Geometry check sheet. Reference: the model listing, model coordinates, mm. Face numbers are marked on the shaded views. A direction names the side the tool comes from. Coordinates: 2 decimals unless noted, no trailing zeros. One line per question, with ' | ' between items.
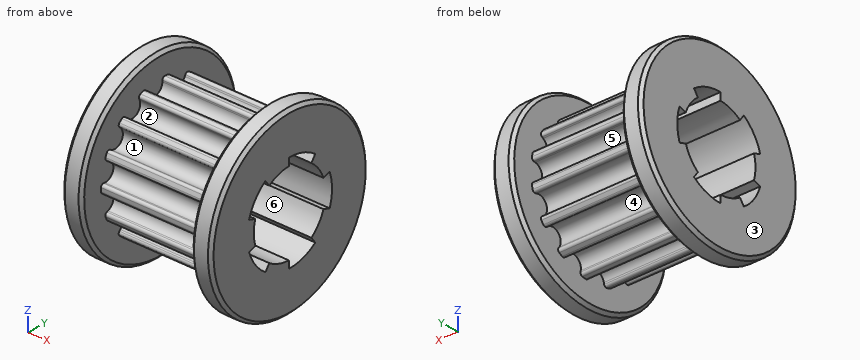
from build123d import *

# Parameters (mm, degrees)
CHAMFER_1_SIZE           = 1
SKETCH_4_W               = 2
SKETCH_4_H               = 1.440270842
CUT_EXTRUDE_1_DEPTH      = 23.179036994
CUT_EXTRUDE_2_REACH      = 24.179
PATTERN_CIRCULAR_3_COUNT = 15
SKETCH_7_R               = 3
CUT_EXTRUDE_3_DEPTH      = 23.173117564
EXTRUDE_START            = 2
SKETCH_9_R               = 9
SKETCH_9_R_2             = 3
EXTRUDE_1_DEPTH          = 2
SKETCH_10_R              = 9
SKETCH_10_R_2            = 3
EXTRUDE_2_DEPTH          = 2
CHAMFER_2_SIZE           = 0.3
SKETCH_11_R              = 4
CUT_EXTRUDE_4_DEPTH      = 20.672315573
CUT_EXTRUDE_5_DEPTH      = 20.672315573
PATTERN_CIRCULAR_4_COUNT = 5
CUT_EXTRUDE_6_DEPTH      = 20.672315573


with BuildPart() as part:
    # Sketch 1 → Revolve 1 (revolve)
    with BuildSketch(Plane.XY, mode=Mode.PRIVATE) as revolve_1_sk:
        Polygon((0, 1.3558), (0, 6.779), (11, 6.779), (11, 2.7116), (20, 2.7116), (20, 1.3558), align=None)
    revolve(revolve_1_sk.sketch.rotate(Axis((0, 0, 0), (1, 0, 0)), 90), axis=Axis((0, 0, 0), (1, 0, 0)))

    # Chamfer 1
    chamfer_1_edges = [part.edges().sort_by_distance(p)[0] for p in [
        (20, 0, -1.3558),
        (0, 0, -1.3558),
    ]]
    chamfer(chamfer_1_edges, length=CHAMFER_1_SIZE)

    # Sketch 4 → Cut-Extrude 1 (cut, through all)
    with BuildSketch(Plane.ZY):
        with Locations((0, 1.635664579)):
            Rectangle(SKETCH_4_W, SKETCH_4_H)
    extrude(amount=-CUT_EXTRUDE_1_DEPTH, mode=Mode.SUBTRACT)

    # Sketch 6 → Cut-Extrude 2 (cut, up to next)
    with BuildSketch(Plane(origin=(0, 0, 0), x_dir=(0, 0, -1), z_dir=(1, 0, 0)), mode=Mode.PRIVATE) as cut_extrude_2_sk1:
        with BuildLine():
            Line((0.921029279, 6.443168288), (0.903216998, 6.298098898))
            ThreePointArc((0.903216998, 6.298098898), (0, 5.499), (-0.903216998, 6.298098898))
            Line((-0.903216998, 6.298098898), (-0.921029279, 6.443168288))
            ThreePointArc((-0.921029279, 6.443168288), (-1.025205225, 6.62105106), (-1.226117469, 6.667194084))
            ThreePointArc((-1.226117469, 6.667194084), (-1.353747907, 6.642454938), (-1.480880455, 6.615272789))
            Line((-1.480880455, 6.615272789), (-1.677528444, 8.216842132))
            ThreePointArc((-1.677528444, 8.216842132), (0, 8.386333901), (1.677528444, 8.216842132))
            Line((1.677528444, 8.216842132), (1.480880455, 6.615272789))
            ThreePointArc((1.480880455, 6.615272789), (1.353747907, 6.642454938), (1.226117469, 6.667194084))
            ThreePointArc((1.226117469, 6.667194084), (1.025205225, 6.62105106), (0.921029279, 6.443168288))
        make_face()
    cut_extrude_2_tool1 = extrude(cut_extrude_2_sk1.sketch, amount=CUT_EXTRUDE_2_REACH, mode=Mode.PRIVATE) & part.part
    cut_extrude_2 = cut_extrude_2_tool1.solids().sort_by_distance((0, 7.172733, 0))[0]
    add(cut_extrude_2, mode=Mode.SUBTRACT)

    # Pattern Circular 3: Cut-Extrude 2 ×15 about axis
    pattern_circular_3_axis = Axis((0, 0, 0), (1, 0, 0))
    for i in range(1, PATTERN_CIRCULAR_3_COUNT):
        add(cut_extrude_2.rotate(pattern_circular_3_axis, i * 360 / PATTERN_CIRCULAR_3_COUNT), mode=Mode.SUBTRACT)

    # Sketch 7 → Cut-Extrude 3 (cut, through all)
    with BuildSketch(Plane.ZY):
        Circle(SKETCH_7_R)
    extrude(amount=-CUT_EXTRUDE_3_DEPTH, mode=Mode.SUBTRACT)

    # Sketch 9 → Extrude 1 (add)
    with BuildSketch(Plane.ZY.offset(EXTRUDE_START)):
        Circle(SKETCH_9_R)
        Circle(SKETCH_9_R_2, mode=Mode.SUBTRACT)
    extrude(amount=-EXTRUDE_1_DEPTH)

    # Sketch 10 → Extrude 2 (add)
    with BuildSketch(Plane(origin=(11, 0, 0), x_dir=(0, 0, -1), z_dir=(1, 0, 0))):
        with Locations(Location((0, 0, 0), (0, 0, 180))):
            Circle(SKETCH_10_R)
        with Locations(Location((0, 0, 0), (0, 0, 180))):
            Circle(SKETCH_10_R_2, mode=Mode.SUBTRACT)
    extrude(amount=EXTRUDE_2_DEPTH)

    # Chamfer 2
    chamfer_2_edges = [part.edges().sort_by_distance(p)[0] for p in [
        (-2, 0, -9),
        (0, 0, -9),
        (13, 0, -9),
        (11, 0, -9),
    ]]
    chamfer(chamfer_2_edges, length=CHAMFER_2_SIZE)

    # Sketch 11 → Cut-Extrude 4 (cut, through all)
    with BuildSketch(Plane.ZY.offset(2)):
        Circle(SKETCH_11_R)
    extrude(amount=-CUT_EXTRUDE_4_DEPTH, mode=Mode.SUBTRACT)

    # Sketch 12 → Cut-Extrude 5 (cut, through all)
    with BuildSketch(Plane.ZY.offset(2)):
        with BuildLine():
            Line((-1.467830723, 4.517518452), (-1.236067977, 3.804226065))
            ThreePointArc((-1.236067977, 3.804226065), (0, 4), (1.236067977, 3.804226065))
            Line((1.236067977, 3.804226065), (1.467830723, 4.517518452))
            ThreePointArc((1.467830723, 4.517518452), (0, 4.75), (-1.467830723, 4.517518452))
        make_face()
    cut_extrude_5 = extrude(amount=-CUT_EXTRUDE_5_DEPTH, mode=Mode.SUBTRACT)

    # Pattern Circular 4: Cut-Extrude 5 ×5 about axis
    pattern_circular_4_axis = Axis((0, 0, 0), (1, 0, 0))
    for i in range(1, PATTERN_CIRCULAR_4_COUNT):
        add(cut_extrude_5.rotate(pattern_circular_4_axis, i * 360 / PATTERN_CIRCULAR_4_COUNT), mode=Mode.SUBTRACT)

    # Sketch 13 → Cut-Extrude 6 (cut, through all)
    with BuildSketch(Plane.ZY.offset(2)):
        with BuildLine():
            Line((-1.593519466, 4.58074183), (-1.361698423, 3.86727002))
            ThreePointArc((-1.361698423, 3.86727002), (-2.409919534, 3.316969677), (-3.257204399, 2.490104316))
            Line((-3.257204399, 2.490104316), (-3.864119771, 2.931054144))
            ThreePointArc((-3.864119771, 2.931054144), (-4.612624104, 1.498732423), (-4.848968963, -0.1))
            Line((-4.848968963, -0.1), (-4.098780306, -0.1))
            ThreePointArc((-4.098780306, -0.1), (-3.899331717, -1.266969677), (-3.374761449, -2.328300917))
            Line((-3.374761449, -2.328300917), (-3.981676821, -2.769250746))
            ThreePointArc((-3.981676821, -2.769250746), (-2.850758474, -3.923732423), (-1.403308163, -4.642545229))
            Line((-1.403308163, -4.642545229), (-1.171487119, -3.929073419))
            ThreePointArc((-1.171487119, -3.929073419), (0, -4.1), (1.171487119, -3.929073419))
            Line((1.171487119, -3.929073419), (1.403308163, -4.642545229))
            ThreePointArc((1.403308163, -4.642545229), (2.850758474, -3.923732423), (3.981676821, -2.769250746))
            Line((3.981676821, -2.769250746), (3.374761449, -2.328300917))
            ThreePointArc((3.374761449, -2.328300917), (3.899331717, -1.266969677), (4.098780306, -0.1))
            Line((4.098780306, -0.1), (4.848968963, -0.1))
            ThreePointArc((4.848968963, -0.1), (4.612624104, 1.498732423), (3.864119771, 2.931054144))
            Line((3.864119771, 2.931054144), (3.257204399, 2.490104316))
            ThreePointArc((3.257204399, 2.490104316), (2.409919534, 3.316969677), (1.361698423, 3.86727002))
            Line((1.361698423, 3.86727002), (1.593519466, 4.58074183))
            ThreePointArc((1.593519466, 4.58074183), (0, 4.85), (-1.593519466, 4.58074183))
        make_face()
    extrude(amount=-CUT_EXTRUDE_6_DEPTH, mode=Mode.SUBTRACT)


solid = part.part
1. Go/stop test with flat-tipped pins: P1, Ø0.8, axis at x = 4, z = 4.5, coming from the +Y side; P2, Ø3, axis at x = 6.5, y = -3, coming from the +Z side; P3, Ø8, axis at x = 5, y = 3.5, coming from the -Z side. Record where each tip stops, or that it passes through.
Worked answers:
P1: y = 5.4 | P2: z = 6.51 | P3: z = -6.76
2. Tool access check on the marked faces 4, 5 and 6. Record the directions out of +Z, -Z, +X, -X, +Y, -Y that give a thin tool (end or side, any length) a straight path to the whole face; none if there is none.
Worked answers:
face 4: none | face 5: +Y | face 6: +X, -X
3. Material ranges on line 1 (Y direction, x = 11.75, z = 0); line 2 (Y direction, x = 5.5, z = 0); line 3 (X direction, y = 4, z = -4.25), recorded low to high. Write a range as from..to.
Worked answers:
line 1: -9..-4.1, 4.85..9 | line 2: -6.78..-4.1, 4.85..5.5 | line 3: -2..0, 11..13
4. Mould release check, pull along Z, two halves, no side actions. Record for the marked faces 1, 2 and 3: released by +Z, released by -Z, zero draft, split by the parting line, or undercut.
Worked answers:
face 1: undercut | face 2: undercut | face 3: zero draft
